Answer from the drawing. Dimensions are ordinates in mm from the lowest x, y and z of the part. Round coordinates to 2 decimals unless told otherwise and drop trailing zeros. Write each loop counter-clockwise with the first axis right and the second up, starting at its lowest first coordinate (ties: lowest second). Pieces come first, ordered by that corner, then holes.
1. Flat-ended cylindrical pins translate along their axes: pin 1 Ø5 at (y, z) = (8, 5.5) entering from +X; pin 2 Ø1.4 at (x, y) = (10, 8) entering from +Z; pin 3 Ø4 at (x, z) = (25.5, 9) entering from -Y. Find the tip coordinate at first contact, or state that the pin passes through.
2. Find section D-D (z = 4). Write down the section's boundary in (x, y).
3. Straight lines are drawn through the part: probe 1 along X at (y, z) = (8, 9.65); probe 2 along Y at (x, z) = (10, 8.3); probe 3 along Y at (x, z) = (25, 7.55). For each, find the intervals that lie inside material, in ascending order.
4. Find section C-C (x = 10). Write down the section's boundary in (y, z), and give its area (3 significant figures).
5. Determine the mould class of the marked faces 1 and 2 for opening direction X: pulls with the +X half, pulls with the -X half, needs draft (parallel to the pull), parting line crosses it, or undercut.
6. Find section B-B (y = 8). Write down the section's boundary in (x, z), and give its area (3 significant figures).
7. Find section A-A (z = 8.5). Write down the section's boundary in (x, y).
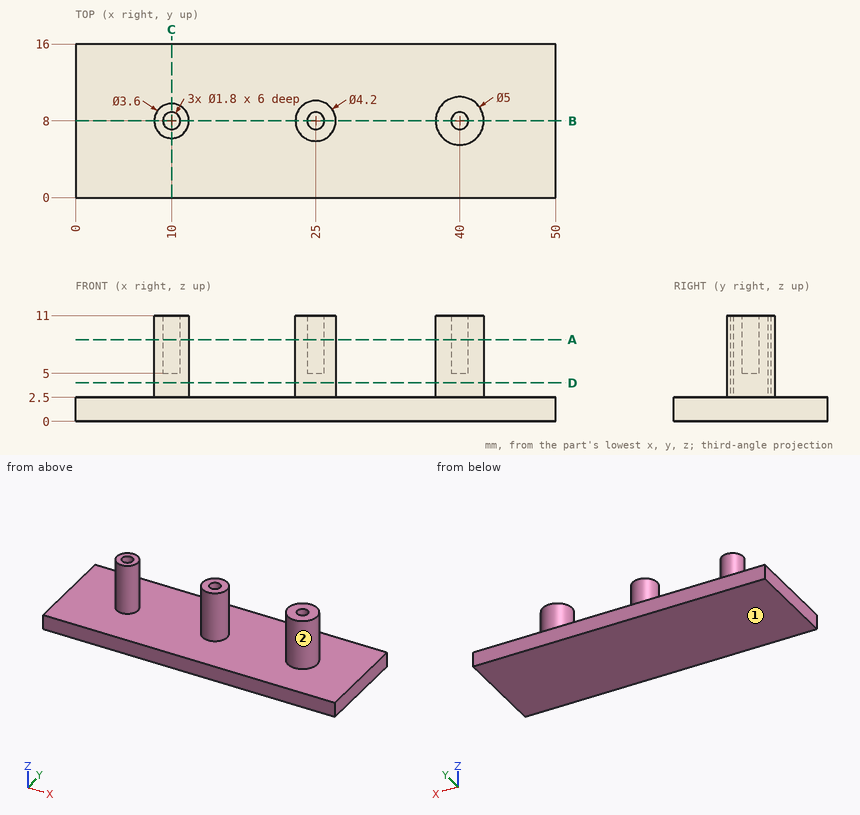
Worked answers:
1. pin 1: stops at x = 42.5
1. pin 2: stops at z = 5
1. pin 3: stops at y = 5.9
2. outline: circle Ø3.6 at (10, 8); circle Ø4.2 at (25, 8); circle Ø5 at (40, 8)
3. probe 1: x = 8.2 to 9.1, 10.9 to 11.8, 22.9 to 24.1, 25.9 to 27.1, 37.5 to 39.1, 40.9 to 42.5
3. probe 2: y = 6.2 to 7.1, 8.9 to 9.8
3. probe 3: y = 5.9 to 7.1, 8.9 to 10.1
4. outline: (0, 0) - (16, 0) - (16, 2.5) - (9.8, 2.5) - (9.8, 11) - (8.9, 11) - (8.9, 5) - (7.1, 5) - (7.1, 11) - (6.2, 11) - (6.2, 2.5) - (0, 2.5) - close
4. area: 59.8 mm2
5. face 1: needs draft
5. face 2: undercut
6. outline: (0, 0) - (50, 0) - (50, 2.5) - (42.5, 2.5) - (42.5, 11) - (40.9, 11) - (40.9, 5) - (39.1, 5) - (39.1, 11) - (37.5, 11) - (37.5, 2.5) - (27.1, 2.5) - (27.1, 11) - (25.9, 11) - (25.9, 5) - (24.1, 5) - (24.1, 11) - (22.9, 11) - (22.9, 2.5) - (11.8, 2.5) - (11.8, 11) - (10.9, 11) - (10.9, 5) - (9.1, 5) - (9.1, 11) - (8.2, 11) - (8.2, 2.5) - (0, 2.5) - close
6. area: 201 mm2
7. outline: circle Ø3.6 at (10, 8); circle Ø4.2 at (25, 8); circle Ø5 at (40, 8); hole circle Ø1.8 at (10, 8); hole circle Ø1.8 at (25, 8); hole circle Ø1.8 at (40, 8)
